from build123d import *

# Parameters (mm, degrees)
EXTRUDE_1_DEPTH     = 3
EXTRUDE_START       = -120
EXTRUDE_2_OUTLINE_R = 1.5
EXTRUDE_2_DEPTH     = 118


# Read off the part's stored shape, not the designer's step: 凸台-拉伸2
with BuildPart() as part:
    # 草图1 → 凸台-拉伸1 (new body)
    with BuildSketch(Plane.XY):
        with BuildLine():
            Line((10, -29.761156884), (10, -59.761156884))
            ThreePointArc((10, -59.761156884), (4, -65.761156884), (-2, -59.761156884))
            Line((-2, -59.761156884), (-2, -29.761156884))
            ThreePointArc((-2, -29.761156884), (4, -23.761156884), (10, -29.761156884))
        make_face()
        with BuildLine():
            Line((0, -29.761156884), (0, -59.761156884))
            ThreePointArc((0, -59.761156884), (4, -63.761156884), (8, -59.761156884))
            Line((8, -59.761156884), (8, -29.761156884))
            ThreePointArc((8, -29.761156884), (4, -25.761156884), (0, -29.761156884))
        make_face(mode=Mode.SUBTRACT)
    extrude(amount=EXTRUDE_1_DEPTH)

    # 凸台-拉伸2 outline → 凸台-拉伸2 (add)
    with BuildSketch(Plane.YZ.offset(EXTRUDE_START)):
        with Locations((-44.761156884, 1.5)):
            Circle(EXTRUDE_2_OUTLINE_R)
    extrude(amount=EXTRUDE_2_DEPTH)


solid = part.part
The listing builds one solid part. Answer for the finished solid, in the listing's coordinates (mm). A direction names the side the tool comes from. Round coordinates to 2 decimals unless told otherwise and drop trailing zeros. Order: outer loops, then holes, each group sorted by start corner. A loop starts at its lowest first (then second) coordinate and runs counter-clockwise, first axis right, second up. Notation, with made-up numbers: M 8.25,30.5 L 27.25,30.5 A32 ccw 27.25,68.5 Z; hole C -3.75,44.5 d5. An arc over 180 degrees is marked long. Answer in a Markdown table with one row per item. Add a question column.
1) Which of the six approach directions +Z, -Z, +X, -X, +Y, -Y give full straight-line access (tool end or side, diameter ignored) to faces 4 (the face through (3.91, -63.76, 1.48)), 5 (the face through (9, -44, 3)), 6 (the face through (-61.83, -43.33, 1.95))?
2) Flat-ended cylindrical pins translate along their axes: pin 1 Ø0.9 at (y, z) = (-40, 2) entering from -X; pin 2 Ø1 at (x, z) = (-104, 1) entering from -Y; pin 3 Ø1.5 at (y, z) = (-61.5, 0.5) entering from +X. Find the tip coordinate at first contact, or state that the pin passes through.
3) The part is cut by section B-B on x = 4. Determine the outline of the cut face in (y, z), plus the area to 3 significant figures.
4) The part is cut by section C-C on z = 1.5. Determine the outline of the cut face in (x, y), plus the area to 3 significant figures.
5) Consider line 1 along Y through (x, z) = (4, 1.65); line 2 along X through (y, z) = (-32.5, 2.35); line 3 along Y through (x, z) = (-111, 1.4). Determine where each line is inside the solid, lowest interval first. Write a range as from..to.
6) The part is cut by section A-A on y = -55. Determine the outline of the cut face in (x, z).
7) Determine the mould class of faces 1 (the face through (0, -45, 1)), 2 (the face through (3.868, -23.763, 1.479)), 3 (the face through (9, -44, 0)) for opening direction Y: pulls with the +Y half, pulls with the -Y half, needs draft (parallel to the pull), parting line crosses it, or undercut.
Findings below:
| question | item | result |
|---|---|---|
| 1 | face 4 | +Z, -Z |
| 1 | face 5 | +Z, +X, -X, +Y, -Y |
| 1 | face 6 | -X |
| 2 | pin 1 | stops at x = -2 |
| 2 | pin 2 | stops at y = -46.26 |
| 2 | pin 3 | stops at x = 9.92 |
| 3 | outline | M -65.76,0 L -63.76,0 L -63.76,3 L -65.76,3 Z; M -25.76,0 L -23.76,0 L -23.76,3 L -25.76,3 Z |
| 3 | area | 12.0 mm² |
| 4 | outline | M -120,-46.26 L -2,-46.26 L -2,-59.76 A6 ccw 10,-59.76 L 10,-29.76 A6 ccw -2,-29.76 L -2,-43.26 L -120,-43.26 Z; hole M 0,-59.76 A4 ccw 8,-59.76 L 8,-29.76 A4 ccw 0,-29.76 Z |
| 4 | area | 537 mm² |
| 5 | line 1 | y = -65.76..-63.76, -25.76..-23.76 |
| 5 | line 2 | x = -2..0, 8..10 |
| 5 | line 3 | y = -46.26..-43.26 |
| 6 | outline | M -2,0 L 0,0 L 0,3 L -2,3 Z; M 8,0 L 10,0 L 10,3 L 8,3 Z |
| 7 | face 1 | undercut |
| 7 | face 2 | pulls with the +Y half |
| 7 | face 3 | needs draft |
